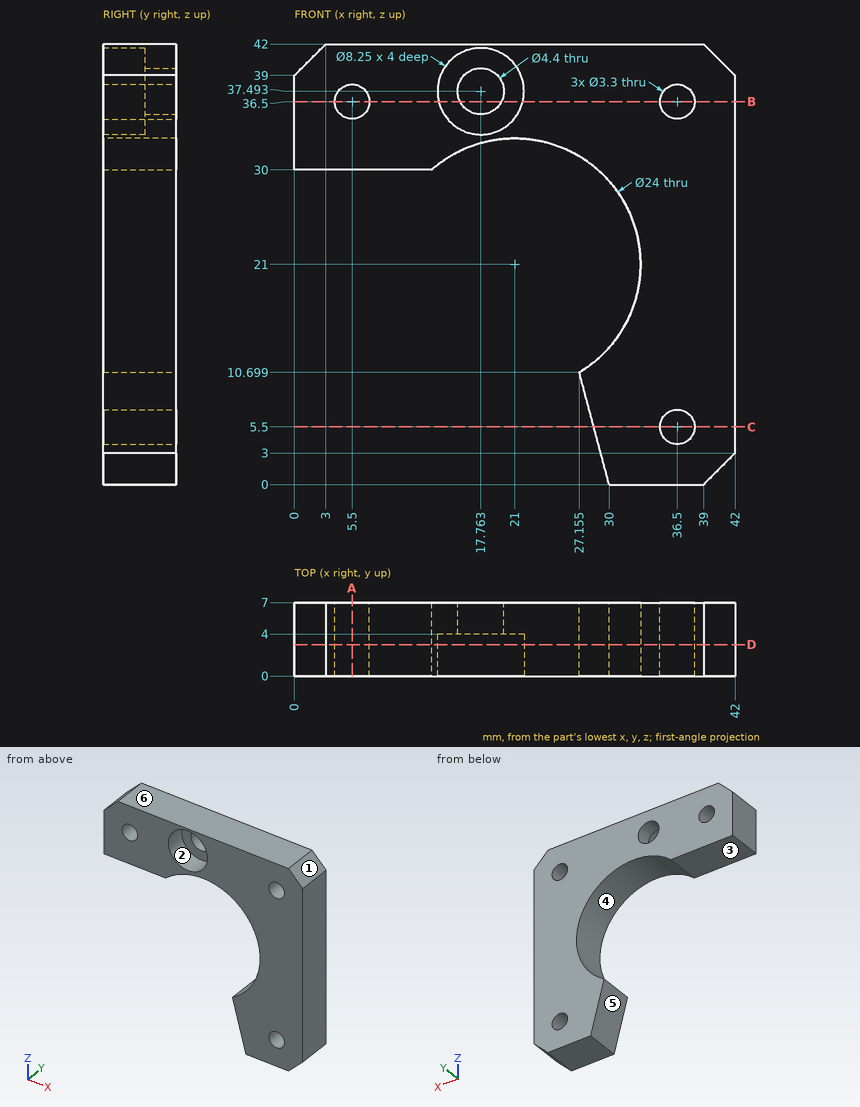
Design review of the part shown in the three views and the two pictorial views. Dimensions are in mm from the part's minimum x, y and z. A direction names the side the tool comes from. Give positions to 0.01 mm unless a question says otherwise; leave off trailing zeros. Loops run counter-clockwise (first coordinate to the right, second up) from the corner with the lowest first, then second, coordinate; pieces in that order, holes last. Notation, with made-up numbers: (67, 20.5) - (79, 20.5) arc R7 cw to (79, 27.5) - close; hole circle Ø11 at (-2.5, 6.25). An arc over 180 degrees is marked (long way). Use CSV: the item, a comma, the result in double quotes. Start each with the question number.
1. Wall thickness on L1, parallel to Z at x = 36.5, y = 3; L2, parallel to Z at x = 4.5, y = 4.25; L3, parallel to Z at x = 5.5, y = 2.5: over which ranges is each line inside the solid? List them lowest first.
2. Add section B-B (z = 36.5). State the section outline as (x, y) points, plus the area to 3 significant figures.
3. Add section C-C (z = 5.5). State the section outline as (x, y) points.
4. Machinability: for the marked faces 1, 2 and 3, which of the approach directions +Z, -Z, +X, -X, +Y, -Y give a long, thin tool a straight path to every point of the face, cutting with its end or side? Answer none if there is none.
5. Insertion check: P1, Ø1.5, axis at x = 14.5, y = 1.5, coming from the -Z side. The pin has a flat end and moves straight along its axis. Give the tip position at first contact, or say it passes through.
6. Add section D-D (y = 3). Count the separate pieces of the cut face and the enclosed holes in it, plus the area to 3 significant figures.
7. Draft analysis for pull direction X (two halves, no side actions). For the marked faces 4, 5 and 6, state which applies: released by +X, released by -X, zero draft, split by the parting line, or undercut.
8. Add section A-A (x = 5.5). State the section outline as (y, z) points.
Results found:
1,L1,"z = 0 to 3.85, 7.15 to 34.85, 38.15 to 42"
1,L2,"z = 30 to 35.19, 37.81 to 42"
1,L3,"z = 30 to 34.85, 38.15 to 42"
2,outline,"(0, 0) - (3.85, 0) - (3.85, 7) - (0, 7) - close; (7.15, 0) - (13.76, 0) - (13.76, 4) - (15.8, 4) - (15.8, 7) - (7.15, 7) - close; (19.73, 4) - (21.77, 4) - (21.77, 0) - (34.85, 0) - (34.85, 7) - (19.73, 7) - close; (38.15, 0) - (42, 0) - (42, 7) - (38.15, 7) - close"
2,area,"204 mm²"
3,outline,"(28.54, 0) - (34.85, 0) - (34.85, 7) - (28.54, 7) - close; (38.15, 0) - (42, 0) - (42, 7) - (38.15, 7) - close"
4,face 1,"+Z, +X, +Y, -Y"
4,face 2,"-Y"
4,face 3,"-Z, -X, +Y, -Y"
5,P1,"stops at z = 30.56"
6,separate pieces,"1"
6,enclosed holes,"4"
6,area,"725 mm²"
7,face 4,"undercut"
7,face 5,"released by -X"
7,face 6,"zero draft"
8,outline,"(0, 30) - (7, 30) - (7, 34.85) - (0, 34.85) - close; (0, 38.15) - (7, 38.15) - (7, 42) - (0, 42) - close"
